```python
from build123d import *
from build123d import SkipClean  # not in build123d's __all__

# Parameters (mm, degrees)
F0_W     = 99.2605239153
F0_H     = 106.7802645266
F1_DEPTH = 59.944
F3_DEPTH = 99.2615239153
F5_DEPTH = 14.224
F7_DEPTH = 10.922
F8_R     = 11.0925650774
F8_R_2   = 12.2440148534
F9_DEPTH = 106.7812645266


# Not quite as in the source:
# - after a boolean that leaves OpenCascade's solid faulty, fix() repairs it


with BuildPart() as f1:
    # F0 (on Front) → F1 (new body, symmetric)
    with BuildSketch(Plane.XZ):
        with Locations((5.4142102599, -9.7756590694)):
            Rectangle(F0_W, F0_H)
    extrude(amount=F1_DEPTH, both=True)

    # F2 (on face) → F3 (cut, through all)
    with BuildSketch(Plane.YZ.offset(55.0444722176)):
        with BuildLine():
            Line((23.4615784138, 43.6144731939), (-17.1450003982, 43.6144731939))
            ThreePointArc((-17.1450003982, 43.6144731939), (3.1582890078, 21.4579654327), (23.4615784138, 43.6144731939))
        make_face()
    extrude(amount=-F3_DEPTH, mode=Mode.SUBTRACT)

    # F4 (on face) → F5 (join)
    with BuildSketch(Plane.YZ.offset(55.0444722176)):
        with BuildLine():
            Line((-17.1450003982, 43.6144731939), (-24.3639480323, 43.6144731939))
            ThreePointArc((-24.3639480323, 43.6144731939), (2.5567095727, 13.9394518293), (29.4773671776, 43.6144731939))
            Line((29.4773671776, 43.6144731939), (23.4615784138, 43.6144731939))
            ThreePointArc((23.4615784138, 43.6144731939), (3.1582890078, 21.4579654327), (-17.1450003982, 43.6144731939))
        make_face()
    with SkipClean():  # cleaning this boolean's faces spoils the solid; the shape is the same uncleaned
        extrude(amount=F5_DEPTH)

    # F6 (on face) → F7 (join)
    with BuildSketch(Plane(origin=(-44.2160516977, 0, 0), x_dir=(0, -1, 0), z_dir=(-1, 0, 0))):
        with BuildLine():
            Line((-23.4615784138, 43.6144731939), (-28.8757905364, 43.6144731939))
            ThreePointArc((-28.8757905364, 43.6144731939), (-2.8575006872, 14.036395677), (23.1607891619, 43.6144731939))
            Line((23.1607891619, 43.6144731939), (17.1450003982, 43.6144731939))
            ThreePointArc((17.1450003982, 43.6144731939), (-3.1582890078, 21.4579654327), (-23.4615784138, 43.6144731939))
        make_face()
    extrude(amount=F7_DEPTH)

    add(f1.part.fix(), mode=Mode.REPLACE)

    # F8 (on face) → F9 (cut, through all)
    with BuildSketch(Plane.XY.offset(43.6144731939)):
        with Locations((5.7150018401, 42.1105287969)):
            Circle(F8_R)
        with Locations((10.2268429473, -40.3057895601)):
            Circle(F8_R_2)
    extrude(amount=-F9_DEPTH, mode=Mode.SUBTRACT)


solid = f1.part
```
Geometry check sheet. Reference: the model listing, model coordinates, mm. Coordinates: 2 decimals unless noted, no trailing zeros. Order: outer loops, then holes, each group sorted by start corner. A loop starts at its lowest first (then second) coordinate and runs counter-clockwise, first axis right, second up. Notation, with made-up numbers: (-3, 79) - (2, 79) arc R20 cw to (2, 97) - close; hole circle Ø9 at (31, 36.5). An arc over 180 degrees is marked (long way). Answer as a JSON object with one key per item and string values. Group by question number.
Item 1: Sectioned sample at B-B, the plane x = 4. Record the cut outline in (y, z) (3 decimals).
Item 2: Sectioned sample at C-C, the plane z = -45.5. Record the cut outline in (x, y) (3 decimals), and give its area (3 significant figures).
Item 3: Sectioned sample at D-D, the plane x = 46. Record the cut outline in (y, z) (3 decimals).
Item 4: Sectioned sample at A-A, the plane y = 37. Record the cut outline in (x, z), and give its area (3 significant figures).
Item 5: Scan lines: probe 1 along X at (y, z) = (42.5, -15); probe 2 along Y at (x, z) = (-32, 28.5); probe 3 along Y at (x, z) = (55.5, 32). Record each from-to range of solid material in increasing order.
Item 6: Draft check along Y on faces 1 (the face through (5, -59.944, -9)), 2 (the face through (0.51, -47.756, -9.028)), 3 (the face through (5, -1, -63.166)), 4 (the face through (5, 59.944, -9)). Enter one of: +Y half, -Y half, draft (parallel to the pull), parting line (faces both ways), or undercut.
Item 7: Depth check by flat-ended pin: pin 1 Ø1.5 at (y, z) = (16, -36) entering from -X. Enter the tip coordinate at first touch or a pass-through.
Resolved:
{
 "1": {"outline": "(-59.944, -63.166) - (-50.848, -63.166) - (-50.848, 43.614) - (-59.944, 43.614) - close; (-29.763, -63.166) - (31.151, -63.166) - (31.151, 43.614) - (23.462, 43.614) arc R20.381 cw (long way) to (-17.145, 43.614) - (-29.763, 43.614) - close; (53.07, -63.166) - (59.944, -63.166) - (59.944, 43.614) - (53.07, 43.614) - close"},
 "2": {"outline": "(-44.216, -59.944) - (55.044, -59.944) - (55.044, 59.944) - (-44.216, 59.944) - close; hole circle Ø22.185 at (5.715, 42.111); hole circle Ø24.488 at (10.227, -40.306)", "area": "11,000 mm^2"},
 "3": {"outline": "(-59.944, -63.166) - (59.944, -63.166) - (59.944, 43.614) - (23.462, 43.614) arc R20.381 cw (long way) to (-17.145, 43.614) - (-59.944, 43.614) - close"},
 "4": {"outline": "(-44.22, -63.17) - (-4.13, -63.17) - (-4.13, 43.61) - (-44.22, 43.61) - close; (15.56, -63.17) - (55.04, -63.17) - (55.04, 43.61) - (15.56, 43.61) - close", "area": "8,500 mm^2"},
 "5": {"probe 1": "-44.22 to -5.37, 16.8 to 55.04", "probe 2": "-59.94 to -12.25, 18.57 to 59.94", "probe 3": "-22.95 to -14.69, 21.01 to 28.07"},
 "6": {"face 1": "-Y half", "face 2": "undercut", "face 3": "draft", "face 4": "+Y half"},
 "7": {"pin 1": "x = -44.22"}
}
